Geometry check sheet. Reference: drawing and pictorial views, mm from the part's lowest x, y, z. Round coordinates to 2 decimals unless told otherwise and drop trailing zeros. Write each loop counter-clockwise with the first axis right and the second up, starting at its lowest first coordinate (ties: lowest second). Pieces come first, ordered by that corner, then holes. Notation, with made-up numbers: M 40.5,62.25 L 54.5,62.25 A20 ccw 54.5,77.25 Z; hole C -24.5,21.5 d3. An arc over 180 degrees is marked long. Answer in a Markdown table with one row per item.
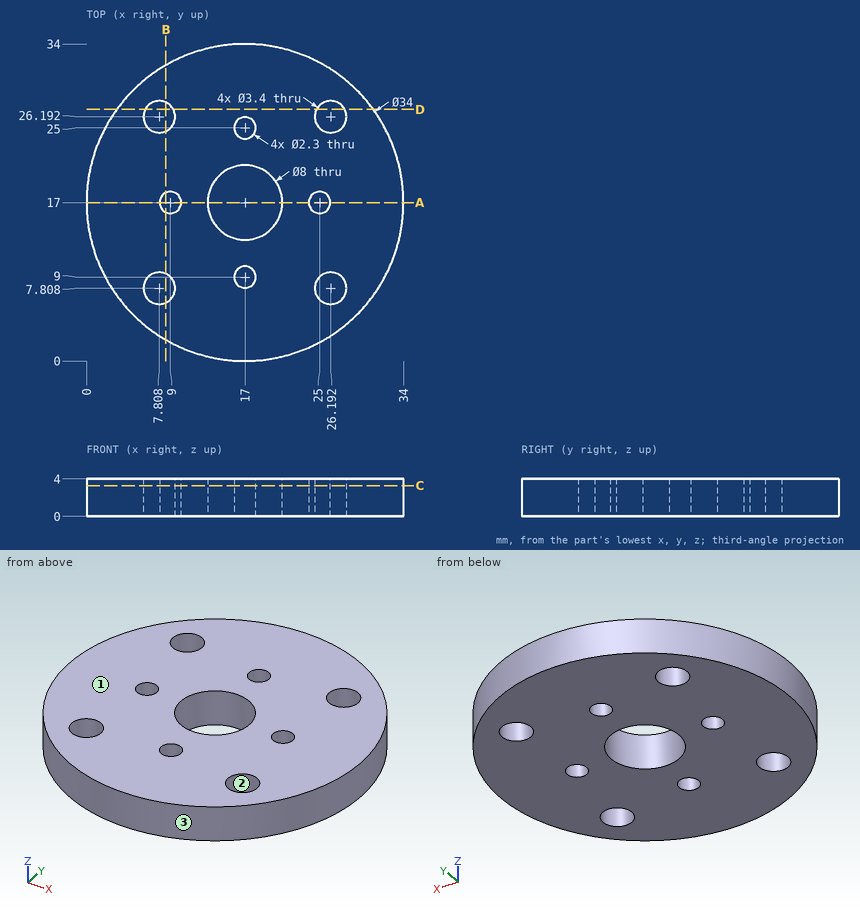
1. Section check C-C, the plane z = 3.3. Count the separate pieces of the cut face and the enclosed holes in it, and give its area (3 significant figures).
Found:
| item | result |
|---|---|
| separate pieces | 1 |
| enclosed holes | 9 |
| area | 805 mm2 |
2. Scan lines: L1, parallel to Y at x = 8.5, z = 0.4 (1 decimal); L2, parallel to Y at x = 27, z = 1.65 (1 decimal). Record each from-to range of solid material in increasing order.
Found:
| item | result |
|---|---|
| L1 | y = 2.3 to 6.3, 9.4 to 16, 18 to 24.6, 27.7 to 31.7 |
| L2 | y = 3.3 to 6.3, 9.3 to 24.7, 27.7 to 30.7 |
3. Section check D-D, the plane y = 27. Record the cut outline in (x, z).
Found:
| item | result |
|---|---|
| outline | M 3.25,0 L 6.31,0 L 6.31,4 L 3.25,4 Z; M 9.3,0 L 24.7,0 L 24.7,4 L 9.3,4 Z; M 27.69,0 L 30.75,0 L 30.75,4 L 27.69,4 Z |
4. Go/stop test with flat-tipped pins: pin 1 (3 mm diameter, centred on x = 7.81, y = 26.19, fed in from +Z); pin 2 (2 mm diameter, centred on x = 20.5, z = 1.5, fed in from +Y) (1 decimal); pin 3 (1.5 mm diameter, centred on x = 3.5, z = 2.5, fed in from -Y) (1 decimal); pin 4 (6 mm diameter, centred on x = 12.5, y = 28.5, fed in from -Z). Record where each tip stops, or that it passes through.
Found:
| item | result |
|---|---|
| pin 1 | passes through |
| pin 2 | stops at y = 33.8 |
| pin 3 | stops at y = 5.8 |
| pin 4 | stops at z = 0 |
5. Draft check along X on the marked faces 1, 2 and 3. Enter one of: +X half, -X half, draft (parallel to the pull), parting line (faces both ways), or undercut.
Found:
| item | result |
|---|---|
| face 1 | draft |
| face 2 | undercut |
| face 3 | parting line |
6. Section check B-B, the plane x = 8.5. Record the cut outline in (y, z) (1 decimal).
Found:
| item | result |
|---|---|
| outline | M 2.3,0 L 6.3,0 L 6.3,4 L 2.3,4 Z; M 9.4,0 L 16,0 L 16,4 L 9.4,4 Z; M 18,0 L 24.6,0 L 24.6,4 L 18,4 Z; M 27.7,0 L 31.7,0 L 31.7,4 L 27.7,4 Z |
7. Section check A-A, the plane y = 17. Record the cut outline in (x, z).
Found:
| item | result |
|---|---|
| outline | M 0,0 L 7.85,0 L 7.85,4 L 0,4 Z; M 10.15,0 L 13,0 L 13,4 L 10.15,4 Z; M 21,0 L 23.85,0 L 23.85,4 L 21,4 Z; M 26.15,0 L 34,0 L 34,4 L 26.15,4 Z |
